from build123d import *

# Parameters (mm, degrees)
SKETCH_1_R          = 3
EXTRUDE_1_DEPTH     = 54
SKETCH_2_R          = 3
SKETCH_2_R_2        = 2.75
CUT_EXTRUDE_1_DEPTH = 0.35


with BuildPart() as part:
    # 스케치1 → 보스-돌출1 (new body)
    with BuildSketch(Plane.XY):
        Circle(SKETCH_1_R)
    extrude(amount=EXTRUDE_1_DEPTH)

    # 스케치2 → 컷-돌출1 (cut, symmetric)
    with BuildSketch(Plane(origin=(0, 0, 1.65), x_dir=(-1, 0, 0), z_dir=(0, 0, -1))):
        Circle(SKETCH_2_R)
        Circle(SKETCH_2_R_2, mode=Mode.SUBTRACT)
    cut_extrude_1 = extrude(amount=CUT_EXTRUDE_1_DEPTH, both=True, mode=Mode.SUBTRACT)

    # 대칭 복사1: 컷-돌출1 across plane
    add(cut_extrude_1.mirror(Plane(origin=(0, 0, 27), x_dir=(1, 0, 0), z_dir=(0, 0, -1))), mode=Mode.SUBTRACT)


solid = part.part
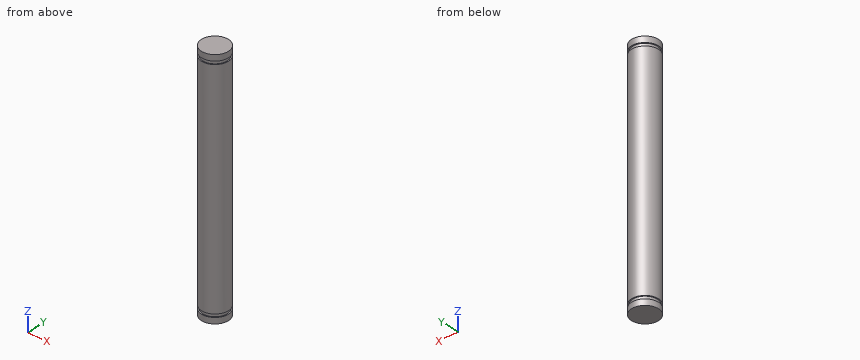
Verification items for the finished model (mm, model axes). Round coordinates to 2 decimals unless told otherwise and drop trailing zeros. Order: outer loops, then holes, each group sorted by start corner. A loop starts at its lowest first (then second) coordinate and runs counter-clockwise, first axis right, second up.
1. Section check C-C on z = 46. Record the cut outline in (x, y), then the cut area to 3 significant figures.
Final values:
outline: circle Ø6 at (0, 0)
area: 28.3 mm2
2. Go/stop test with flat-tipped pins: P1, Ø3, axis at x = -1, z = 39.5, coming from the -Y side; P2, Ø1, axis at x = -1.5, z = 44.5, coming from the -Y side; P3, Ø2, axis at x = -2, z = 7, coming from the +Y side; P4, Ø1, axis at y = -2, z = 39, coming from the -X side. Record where each tip stops, or that it passes through.
Final values:
P1: stops at y = -3
P2: stops at y = -2.83
P3: stops at y = 2.83
P4: stops at x = -2.6
3. Section check B-B on y = 2. Record the cut outline in (x, z).
Final values:
outline: (-2.24, 0) - (2.24, 0) - (2.24, 1.3) - (1.89, 1.3) - (1.89, 2) - (2.24, 2) - (2.24, 52) - (1.89, 52) - (1.89, 52.7) - (2.24, 52.7) - (2.24, 54) - (-2.24, 54) - (-2.24, 52.7) - (-1.89, 52.7) - (-1.89, 52) - (-2.24, 52) - (-2.24, 2) - (-1.89, 2) - (-1.89, 1.3) - (-2.24, 1.3) - close
4. Thickness scan on L1, parallel to Z at x = -2.6, y = -1.15; L2, parallel to Y at x = -2.25, z = 40.5; L3, parallel to Y at x = 0.2, z = 19. Record the ranges inside material, lowest first.
Final values:
L1: z = 0 to 1.3, 2 to 52, 52.7 to 54
L2: y = -1.98 to 1.98
L3: y = -2.99 to 2.99
5. Section check A-A on x = 1.4. Record the cut outline in (y, z), then the cut area to 3 significant figures.
Final values:
outline: (-2.65, 0) - (2.65, 0) - (2.65, 1.3) - (2.37, 1.3) - (2.37, 2) - (2.65, 2) - (2.65, 52) - (2.37, 52) - (2.37, 52.7) - (2.65, 52.7) - (2.65, 54) - (-2.65, 54) - (-2.65, 52.7) - (-2.37, 52.7) - (-2.37, 52) - (-2.65, 52) - (-2.65, 2) - (-2.37, 2) - (-2.37, 1.3) - (-2.65, 1.3) - close
area: 286 mm2
